from build123d import *

# Parameters (mm, degrees)
BOSS_EXTRUDE3_DEPTH = 2
SKETCH4_W           = 46.25
SKETCH4_H           = 27.5
BOSS_EXTRUDE4_DEPTH = 12
FILLET1_R           = 1
FILLET2_R           = 1
FILLET3_R           = 0.25


with BuildPart() as part:
    # Sketch1 → Boss-Extrude3 (new body)
    with BuildSketch(Plane(origin=(0, 0, 0), x_dir=(1, 0, 0), z_dir=(0, 1, 0))):
        with BuildLine():
            Line((33.003141421, 5.895474545), (41.503141421, 1.270474545))
            Line((41.503141421, 1.270474545), (35.611544818, 1.270474545))
            ThreePointArc((35.611544818, 1.270474545), (33.611544818, -0.729525455), (35.611544818, -2.729525455))
            Line((35.611544818, -2.729525455), (41.672555807, -2.729525455))
            Line((41.672555807, -2.729525455), (33.003141421, -7.354525455))
            Line((33.003141421, -7.354525455), (33.003141421, -14.479525455))
            Line((33.003141421, -14.479525455), (-13.246858579, -14.479525455))
            Line((-13.246858579, -14.479525455), (-13.246858579, -7.354525455))
            Line((-13.246858579, -7.354525455), (-21.916272965, -2.729525455))
            Line((-21.916272965, -2.729525455), (-15.855261975, -2.729525455))
            ThreePointArc((-15.855261975, -2.729525455), (-13.855261975, -0.729525455), (-15.855261975, 1.270474545))
            Line((-15.855261975, 1.270474545), (-21.746858579, 1.270474545))
            Line((-21.746858579, 1.270474545), (-13.246858579, 5.895474545))
            Line((-13.246858579, 5.895474545), (-13.246858579, 13.020474545))
            Line((-13.246858579, 13.020474545), (33.003141421, 13.020474545))
            Line((33.003141421, 13.020474545), (33.003141421, 5.895474545))
        make_face()
    extrude(amount=BOSS_EXTRUDE3_DEPTH)

    # Sketch4 → Boss-Extrude4 (add)
    with BuildSketch(Plane.XZ):
        with Locations((9.878141421, 0.729525455)):
            Rectangle(SKETCH4_W, SKETCH4_H)
    extrude(amount=BOSS_EXTRUDE4_DEPTH)

    # Fillet1
    fillet1_edges = [part.edges().sort_by_distance(p)[0] for p in [
        (9.878141421, -12, 14.479525455),
    ]]
    fillet(fillet1_edges, radius=FILLET1_R)

    # Fillet2
    fillet2_edges = [part.edges().sort_by_distance(p)[0] for p in [
        (-13.246858579, -4.5, 14.479525455),
        (33.003141421, -4.5, 14.479525455),
        (33.003141421, -5, -13.020474545),
        (-13.246858579, -5, -13.020474545),
        (9.878141421, -12, -13.020474545),
        (33.003141421, -12, 0.229525455),
        (-13.246858579, -12, 0.229525455),
        (-13.246858579, -11.707106781, 14.186632236),
        (33.003141421, -11.707106781, 14.186632236),
    ]]
    fillet(fillet2_edges, radius=FILLET2_R)

    # Fillet3
    fillet3_edges = [part.edges().sort_by_distance(p)[0] for p in [
        (-21.746858579, 1, -1.270474545),
        (-21.916272965, 1, 2.729525455),
        (41.672555807, 1, 2.729525455),
        (41.503141421, 1, -1.270474545),
    ]]
    fillet(fillet3_edges, radius=FILLET3_R)


solid = part.part
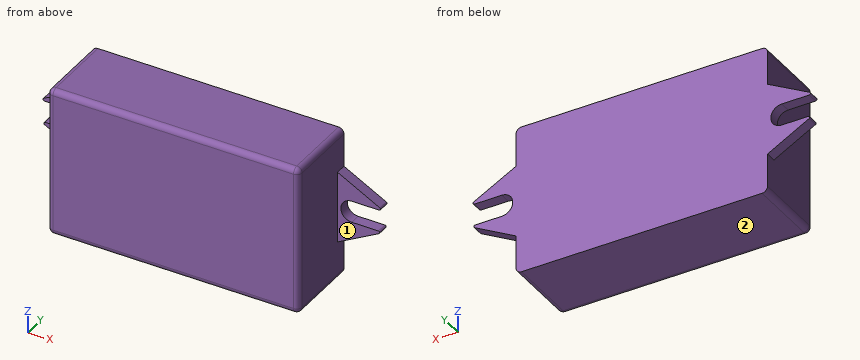
Read the model definition and answer for the solid it produces. Units are mm, in the model's axes. Face numbers are marked on the shaded views. A direction names the side the tool comes from. Round coordinates to 2 decimals unless told otherwise and drop trailing zeros. Write each loop counter-clockwise with the first axis right and the second up, starting at its lowest first coordinate (ties: lowest second). Pieces come first, ordered by that corner, then holes. Notation, with made-up numbers: (26.5, 86) - (37.5, 86) arc R16 cw to (37.5, 92) - close; hole circle Ø1 at (89, 58). An arc over 180 degrees is marked (long way). One line per question, with ' | ' between items. Start each with the question number.
1. For the marked faces 1 and 2, determine the directions among +Z, -Z, +X, -X, +Y, -Y from which every point of the face is accessible in a straight line to the end or side of a thin tool.
2. Each of these flat-tipped pins is pushed along its axis until it touches: pin 1 (1 mm diameter, centred on x = 37, y = 0.5, fed in from +Z); pin 2 (2 mm diameter, centred on y = -5.5, z = -9, fed in from +X); pin 3 (1.6 mm diameter, centred on x = 39.5, y = 1.5, fed in from -Z). Where does it stop, or does it pass through?
3. Section C-C (z = -10.75) is taken. Determine the outline of the cut face in (x, y), and give its area (3 significant figures).
4. Find the intervals of material crossed by probe 1 along X at (y, z) = (0, 10.75); probe 2 along Y at (x, z) = (35, 5); probe 3 along Y at (x, z) = (-12.5, -4.75), in increasing order. Write a range as [from, to].
5. Section A-A (x = -17) is taken. Determine the outline of the cut face in (y, z).
6. Section D-D (y = -5) is taken. Determine the outline of the cut face in (x, z).
7. Section B-B (y = 1) is taken. Determine the outline of the cut face in (x, z), and give its area (3 significant figures).
Filled in:
1) face 1: +Z, -Z, +X, -Y | face 2: -Z, +X, -X, +Y, -Y
2) pin 1: z = 5.49 | pin 2: x = 33 | pin 3: z = -2.8
3) outline: (-13.25, -11) arc R1 ccw to (-12.25, -12) - (32, -12) arc R1 ccw to (33, -11) - (33, 2) - (-13.25, 2) - close | area: 647 mm²
4) probe 1: [-13.25, 33] | probe 2: [0, 2] | probe 3: [-11.97, 2]
5) outline: (0, -3.85) - (2, -3.85) - (2, -1.27) - (0, -1.27) - close; (0, 2.73) - (2, 2.73) - (2, 5.35) - (0, 5.35) - close
6) outline: (-13.25, -12.02) arc R1 ccw to (-12.25, -13.02) - (32, -13.02) arc R1 ccw to (33, -12.02) - (33, 13.48) arc R1 ccw to (32, 14.48) - (-12.25, 14.48) arc R1 ccw to (-13.25, 13.48) - close
7) outline: (-21.03, 3.2) arc R0.25 ccw to (-20.92, 2.73) - (-15.86, 2.73) arc R2 cw to (-15.86, -1.27) - (-20.76, -1.27) arc R0.25 ccw to (-20.88, -1.74) - (-13.25, -5.9) - (-13.25, -12.02) arc R1 ccw to (-12.25, -13.02) - (32, -13.02) arc R1 ccw to (33, -12.02) - (33, -5.9) - (40.64, -1.74) arc R0.25 ccw to (40.52, -1.27) - (35.61, -1.27) arc R2 cw to (35.61, 2.73) - (40.67, 2.73) arc R0.25 ccw to (40.79, 3.2) - (33, 7.35) - (33, 13.48) arc R1 ccw to (32, 14.48) - (-12.25, 14.48) arc R1 ccw to (-13.25, 13.48) - (-13.25, 7.35) - close | area: 1,360 mm²
